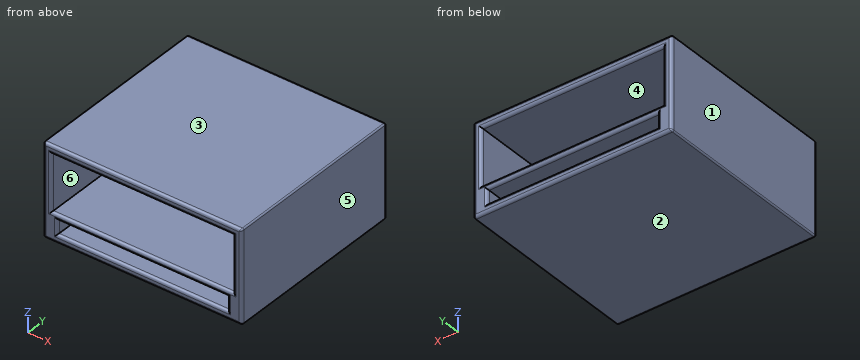
Autodesk Fusion 360 part; units mm, degrees
sketch "Sketch1" plane through (0, 0, 0) normal (0, 0, 1) x (1, 0, 0)
  line L0 (-25, 25) -> (35, 25)
  line L1 (35, 25) -> (35, -27)
  line L2 (35, -27) -> (-25, -27)
  line L3 (-25, -27) -> (-25, 25)
  dimension "d1" = 60
  dimension "d2" = 52
extrude "Extrude1" add sketch "Sketch1" along normal blind 35
extrude "Extrude2" add 1 faces at (-5, 25, 11.6667) along direction (0, 1, 0) blind 5
extrude "Extrude3" add 1 faces at (15, -27, 11.6667) along direction (0, -1, 0) blind 3
extrude "Extrude4" add 1 faces at (35, 10, 11.6667) along direction (1, 0, 0) blind 15
sketch "Sketch2" plane through (0, 30, 0) normal (0, 1, 0) x (-1, 0, 0)
  line L0 (-50, 0) -> (25, 0)
  line L1 (25, 0) -> (25, 35)
  line L2 (25, 35) -> (-50, 35)
  line L3 (-50, 35) -> (-50, 0)
  line L4 (-45, 30) -> (-45, -21)
  line L5 (-45, -21) -> (20, -21)
  line L6 (20, -21) -> (20, 30)
  line L7 (20, 30) -> (-45, 30)
  dimension "d11" = 51
  dimension "d12" = 65
extrude "Extrude5" add 1 faces at (0, -10, 0) along direction (0, 0, -1) blind 30
extrude "Extrude6" cut sketch "Sketch2" against normal blind 59 contours L0 L4 L6 L7
extrude "Extrude7" cut 1 faces at (23.3333, 10.3333, 0) along direction (0, 0, -1) blind 25
extrude "Extrude8" add 1 faces at (0, -10, -30) along direction (0, 0, -1) blind 6
extrude "Extrude9" cut 1 faces at (50, -10, 11.3333) along direction (-1, 0, 0) blind 2
extrude "Extrude10" cut 1 faces at (-25, 10, -12.3333) along direction (1, 0, 0) blind 2
extrude "Extrude11" cut 1 faces at (0.6667, 10, 35) along direction (0, 0, -1) blind 2
extrude "Extrude12" cut 1 faces at (0.6667, -10, -36) along direction (0, 0, 1) blind 3
sketch "Sketch6" plane through (0, 0, 0) normal (0, 1, 0) x (1, 0, 0)
  line L0 (43, 25) -> (43, 28)
  line L1 (45, 28) -> (-20, 28)
  line L2 (-20, 28) -> (-20, 30)
  line L3 (-20, 30) -> (45, 30)
  line L4 (45, 30) -> (45, 28)
  line L5 (30, 30) -> (30, 33)
  dimension "d31" = 3
extrude "Extrude13" cut sketch "Sketch6" along normal blind 30 and the other way blind 38
extrude "Extrude14" add 1 faces at (23.3333, -29, 11.6667) along direction (0, 1, 0) blind 2
sketch "Sketch7" plane through (0, 0, 0) normal (0, 1, 0) x (1, 0, 0)
sketch "Sketch8" plane through (0, 0, 0) normal (0, 1, 0) x (1, 0, 0)
  line L0 (45, 5) -> (-20, 5)
  line L1 (-20, 5) -> (-20, 25)
  line L2 (-20, 25) -> (45, 25)
  line L3 (45, 25) -> (45, 5)
extrude "Extrude15" cut sketch "Sketch8" against normal blind 68
extrude "Extrude16" add 1 faces at (1.6667, 11, 30) along direction (0, 0, -1) blind 10
extrude "Extrude17" cut 1 faces at (0.6667, 10, 33) along direction (0, 0, -1) blind 10
extrude "Extrude18" add 1 faces at (1.6667, 11, 20) along direction (0, 0, -1) blind 0.5
extrude "Extrude19" cut 1 faces at (0.6667, 10, 23) along direction (0, 0, -1) blind 0.5
extrude "Extrude20" add 1 faces at (1.6667, 11, 19.5) along direction (0, 0, -1) blind 1.5
extrude "Extrude21" cut 1 faces at (0.6667, 10, 22.5) along direction (0, 0, -1) blind 0.5
sketch "Sketch9" plane through (0, 0, 0) normal (0, 1, 0) x (1, 0, 0)
extrude "Extrude22" cut 1 faces at (0.6667, 10, 22) along direction (0, 0, -1) blind 1
extrude "Extrude23" add 1 faces at (1.6667, 11, 18) along direction (0, 0, -1) blind 3
extrude "Extrude24" cut 1 faces at (0.6667, 10, 21) along direction (0, 0, -1) blind 3
sketch "Sketch10" plane through (0, 0, 0) normal (0, 1, 0) x (1, 0, 0)
extrude "Extrude25" add 1 faces at (23.3333, -29, -5) along direction (0, 0, -1) blind 8
extrude "Extrude26" add 1 faces at (-22, 30, -13.3333) along direction (0, 1, 0) blind 5
sketch "Sketch11" plane through (0, 35, 0) normal (0, 1, 0) x (-1, 0, 0)
  line L0 (23, 18) -> (-48, 18)
  line L1 (-48, 18) -> (-48, -33)
  line L2 (-48, -33) -> (23, -33)
  line L3 (23, -33) -> (23, 18)
  line L4 (-45, -30) -> (-45, -28)
  line L5 (-45, -28) -> (20, -28)
  line L6 (20, -28) -> (20, -30)
  line L7 (20, -30) -> (-45, -30)
  line L8 (-45, -25) -> (-45, 15)
  line L9 (-45, 15) -> (20, 15)
  line L10 (20, 15) -> (20, -25)
  line L11 (20, -25) -> (-45, -25)
extrude "Extrude27" add sketch "Sketch11" along normal blind 2
extrude "Extrude28" cut 1 faces at (23.3333, -29, -13) along direction (0, 0, 1) blind 5
extrude "Extrude29" cut 1 faces at (23.3333, -29, -8) along direction (0, 0, 1) blind 3
extrude "Extrude30" add 1 faces at (23.3333, -5.6667, 15) along direction (0, 0, -1) blind 15
extrude "Extrude31" cut 1 faces at (24.3333, 14.6667, 18) along direction (0, 0, -1) blind 15
extrude "Extrude32" add 1 faces at (23.3333, -5.6667, 0) along direction (0, 0, -1) blind 5
extrude "Extrude33" cut 1 faces at (24.3333, 14.6667, 3) along direction (0, 0, -1) blind 5
extrude "Extrude34" add 1 faces at (45, 14.6667, -28.6667) along direction (-1, 0, 0) blind 2
extrude "Extrude35" add 1 faces at (-20, -7.6667, -28.6667) along direction (1, 0, 0) blind 2
extrude "Extrude36" cut 1 faces at (22.6667, -7.6667, -28) along direction (0, 0, 1) blind 1
extrude "Extrude37" cut 1 faces at (2.3333, -7.6667, -30) along direction (0, 0, -1) blind 1
extrude "Extrude38" cut 1 faces at (2.3333, -7.6667, -31) along direction (0, 0, -1) blind 1
extrude "Extrude39" add 1 faces at (24.3333, -7.6667, -33) along direction (0, 0, -1) blind 1
extrude "Extrude40" add 1 faces at (24.3333, -7.6667, -34) along direction (0, 0, -1) blind 1
fillet "Fillet1" radius 1 1 faces at (-20.3333, 37, -30.6667)
fillet "Fillet2" radius 1 1 faces at (-20.3333, -30, -30.6667)
fillet "Fillet4" radius 0.5 3 edges at (47.7071, 36.7071, -2.2929) (48, 3.5, -2) (47.7071, -29.7071, -2.2929)
fillet "Fillet5" radius 0.5 3 edges at (47.7071, 36.7071, -34.7071) (48, 3.5, -35) (47.7071, -29.7071, -34.7071)
fillet "Fillet6" radius 0.5 3 edges at (-22.7071, -29.7071, -2.2929) (-23, 3.5, -2) (-22.7071, 36.7071, -2.2929)
fillet "Fillet7" radius 0.5 3 edges at (-22.7071, -29.7071, -34.7071) (-23, 3.5, -35) (-22.7071, 36.7071, -34.7071)
Part model, mm, in its own coordinate system. Face numbers are marked on the shaded views. A direction names the side the tool comes from. Coordinates: 2 decimals unless noted, no trailing zeros. Write each loop counter-clockwise with the first axis right and the second up, starting at its lowest first coordinate (ties: lowest second). Pieces come first, ordered by that corner, then holes.
Item 1: Probe line 1 (Z direction, x = -7, y = 9.5); line 2 (X direction, y = -9.5, z = -20); line 3 (X direction, y = -17.5, z = -30.5). List the from-to ranges inside material, lowest first.
Item 2: Slice it at C-C (x = 33.5). Count the separate pieces of the cut face and the enclosed holes in it, and give its area (3 significant figures).
Item 3: Which spindle directions (+Z, -Z, +X, -X, +Y, -Y) get a long thin tool onto all of the face, cutting with end or side? Do the marked faces 5 and 6. Say none if no direction does.
Item 4: Slice it at D-D (z = -30.5). Write the cut outline in (x, y), and give its area (3 significant figures).
Item 5: Slice it at B-B (y = 2.5). Write the cut outline in (x, z).
Item 6: Mould opens along Z. For the marked faces 1, 2, 3 and 4 say: released by +Z, released by -Z, zero draft, split by the parting line, or undercut.
Item 7: Slice it at A-A (z = -6). Write the cut outline in (x, y).
Results found:
1. line 1: z = -35 to -32, -27 to -25, -5 to -2
1. line 2: x = -23 to -20, 45 to 48
1. line 3: x = -23 to -18, 43 to 48
2. separate pieces: 3
2. enclosed holes: 0
2. area: 533 mm2
3. face 5: +Z, -Z, +X, +Y, -Y
3. face 6: +Y, -Y
4. outline: (-23, -29) arc R1 ccw to (-22, -30) - (-19, -30) arc R1 ccw to (-18, -29) - (-18, 36) arc R1 ccw to (-19, 37) - (-22, 37) arc R1 ccw to (-23, 36) - close; (43, -29) arc R1 ccw to (44, -30) - (47, -30) arc R1 ccw to (48, -29) - (48, 36) arc R1 ccw to (47, 37) - (44, 37) arc R1 ccw to (43, 36) - close
4. area: 668 mm2
5. outline: (-23, -34.5) arc R0.5 ccw to (-22.5, -35) - (47.5, -35) arc R0.5 ccw to (48, -34.5) - (48, -2.5) arc R0.5 ccw to (47.5, -2) - (-22.5, -2) arc R0.5 ccw to (-23, -2.5) - close; hole (-20, -25) - (45, -25) - (45, -5) - (-20, -5) - close; hole (-18, -32) - (43, -32) - (43, -27) - (-18, -27) - close
6. face 1: zero draft
6. face 2: released by -Z
6. face 3: released by +Z
6. face 4: undercut
7. outline: (-23, -29) arc R1 ccw to (-22, -30) - (-21, -30) arc R1 ccw to (-20, -29) - (-20, 36) arc R1 ccw to (-21, 37) - (-22, 37) arc R1 ccw to (-23, 36) - close; (45, -29) arc R1 ccw to (46, -30) - (47, -30) arc R1 ccw to (48, -29) - (48, 36) arc R1 ccw to (47, 37) - (46, 37) arc R1 ccw to (45, 36) - close
